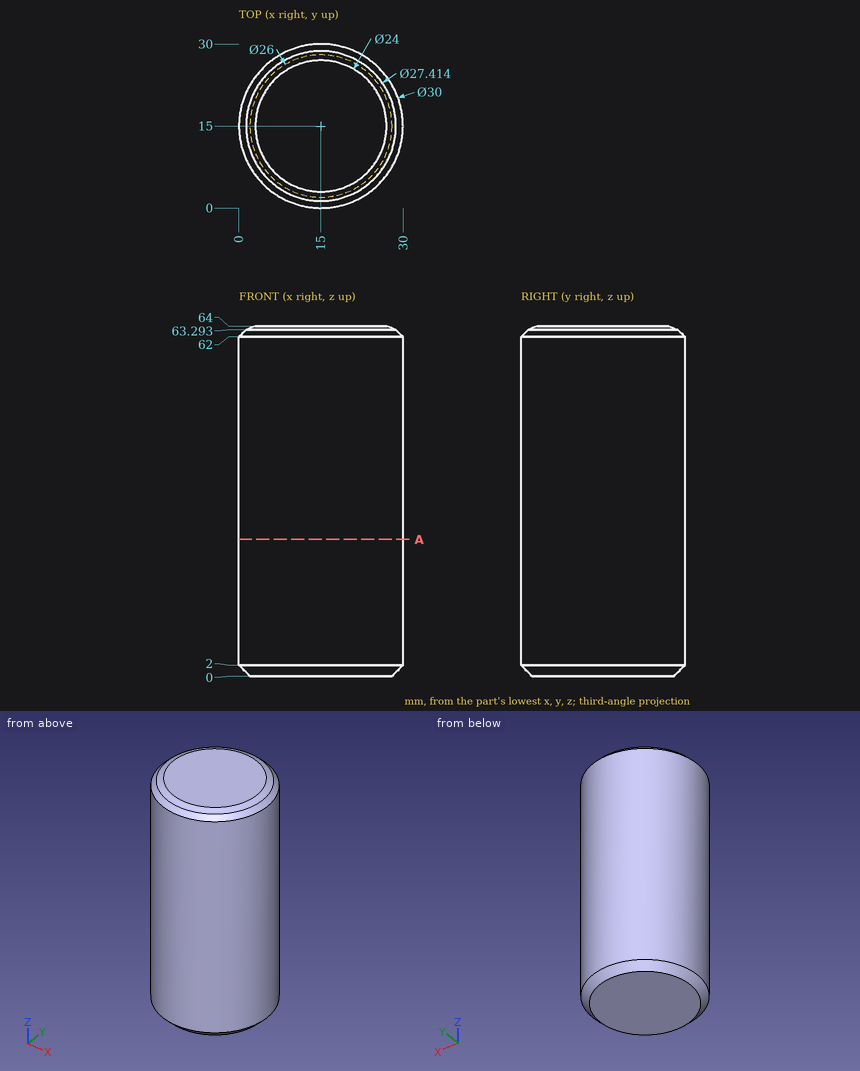
Design review of the part shown in the three views and the two pictorial views. Dimensions are in mm from the part's minimum x, y and z. Round coordinates to 2 decimals unless told otherwise and drop trailing zeros. Order: outer loops, then holes, each group sorted by start corner. A loop starts at its lowest first (then second) coordinate and runs counter-clockwise, first axis right, second up.
(1) Wall thickness on L1, parallel to Y at x = 15.5, z = 56; L2, parallel to X at y = 7.5, z = 36; L3, parallel to X at y = 26.75, z = 26 (1 decimal): over which ranges is each line inside the solid? List them lowest first.
Working result:
L1: y = 0.01 to 29.99
L2: x = 2.01 to 27.99
L3: x = 5.7 to 24.3
(2) Take a section at A-A, the plane z = 25. State the section outline as (x, y) points.
Working result:
outline: circle Ø30 at (15, 15)
(3) For P1, Ø5, axis at x = 9.5, z = 44.5, coming from the +Y side; P2, Ø3, axis at y = 4.5, z = 32, coming from the -X side; P3, Ø4, axis at x = 5.5, z = 31, coming from the -Y side, all flat-tipped, find the tip position at first contact; note any pin that passes through.
Working result:
P1: stops at y = 29.7
P2: stops at x = 3
P3: stops at y = 2.01
